from build123d import *

# Parameters (mm, degrees)
SKETCH1_R           = 1.6
BOSS_EXTRUDE1_DEPTH = 3
FILLET1_R           = 10
FILLET2_R           = 2
FILLET3_R           = 2


# Some blends are built 0.0001 mm under size
with BuildPart() as part:
    # Sketch1 → Boss-Extrude1 (new body)
    with BuildSketch(Plane.XY):
        with BuildLine():
            Line((-15, 37.5), (-11.986741947, -0.333454454))
            Line((-11.986741947, -0.333454454), (-11.77, -31.11))
            ThreePointArc((-11.77, -31.11), (-7.007950772, -32.588761506), (-3.921159912, -36.504827214))
            ThreePointArc((-3.921159912, -36.504827214), (0, -39.2), (3.921159912, -36.504827214))
            ThreePointArc((3.921159912, -36.504827214), (7.007950772, -32.588761506), (11.77, -31.11))
            Line((11.77, -31.11), (11.986741947, -0.333454454))
            Line((11.986741947, -0.333454454), (15, 37.5))
            Line((15, 37.5), (15, 62.5))
            ThreePointArc((15, 62.5), (14.0627417, 64.7627417), (11.8, 65.7))
            Line((11.8, 65.7), (-11.8, 65.7))
            ThreePointArc((-11.8, 65.7), (-14.0627417, 64.7627417), (-15, 62.5))
            Line((-15, 62.5), (-15, 37.5))
        make_face()
        with Locations((7.8, 0)):
            Circle(SKETCH1_R, mode=Mode.SUBTRACT)
        with Locations((-12, 37.5)):
            Circle(SKETCH1_R, mode=Mode.SUBTRACT)
        with Locations((-12, 62.5)):
            Circle(SKETCH1_R, mode=Mode.SUBTRACT)
        Polygon((-7.5, 57.5), (7.5, 57.5), (7.5, 52), (11.5, 52), (11.5, 48), (7.5, 48), (7.5, 42.5), (-7.5, 42.5), (-7.5, 48), (-11.5, 48), (-11.5, 52), (-7.5, 52), align=None, mode=Mode.SUBTRACT)
        with Locations((12, 37.5)):
            Circle(SKETCH1_R, mode=Mode.SUBTRACT)
        with Locations((12, 62.5)):
            Circle(SKETCH1_R, mode=Mode.SUBTRACT)
        with Locations((-7.8, 0)):
            Circle(SKETCH1_R, mode=Mode.SUBTRACT)
        with Locations((0, -35)):
            Circle(SKETCH1_R, mode=Mode.SUBTRACT)
    extrude(amount=BOSS_EXTRUDE1_DEPTH)

    # Fillet1
    # the kernel refuses this fillet: 10 mm, written as the material it adds along each edge
    with BuildSketch(Plane(origin=(-11.986741947, -0.333454454, 0), x_dir=(-0.07939391755808242, 0.9968433206150205, 0), z_dir=(0, 0, 1)), Plane(origin=(11.986741947, -0.333454454, 0), x_dir=(-0.0070422644314045895, -0.9999752029483923, 0), z_dir=(0, 0, 1))) as fillet1_piece_1:
        with BuildLine():
            CenterArc((FILLET1_R * 0.0362334645201, FILLET1_R), FILLET1_R, 265.849766407, 4.150233593)
            Line((-FILLET1_R * 0.0361384500424, FILLET1_R * 0.00262228519856), (0, 0))
            Line((0, 0), (FILLET1_R * 0.0362334645201, 0))
        make_face()
    extrude(amount=3)
    # the kernel refuses this fillet: 10 mm, written as the material it takes off along each edge
    with BuildSketch(Plane(origin=(-11.77, -31.11, -17.521148691), x_dir=(-0.007042264431403126, 0.9999752029483922, 0), z_dir=(0, 0, 1))) as fillet1_2_piece_1:
        with BuildLine():
            CenterArc((7.008459476, -10), FILLET1_R, 90, 56.873561784)
            ThreePointArc((-1.366206899, -4.535115453), (-0.357121593, -2.365760003), (0, 0))
            Line((0, 0), (7.008459476, 0))
        make_face()
    extrude(amount=38.042297381, mode=Mode.SUBTRACT)
    with BuildSketch(Plane(origin=(-15, 37.5, -0.993992828), x_dir=(0, 1, 0), z_dir=(0, 0, 1)), Plane(origin=(15, 37.5, -0.993992828), x_dir=(-0.07939391755808864, -0.9968433206150199, 0), z_dir=(0, 0, 1))) as fillet1_2_piece_2:
        with BuildLine():
            CenterArc((FILLET1_R * 0.0397597131124, -FILLET1_R), FILLET1_R, 90, 4.553728958)
            Line((-FILLET1_R * 0.0396342044457, -FILLET1_R * 0.00315667938498), (0, 0))
            Line((0, 0), (FILLET1_R * 0.0397597131124, 0))
        make_face()
    extrude(amount=4.987985656, mode=Mode.SUBTRACT)
    with BuildSketch(Plane(origin=(11.77, -31.11, -17.521148691), x_dir=(-0.9595036182786473, -0.2816963019107352, 0), z_dir=(0, 0, 1))) as fillet1_2_piece_3:
        with BuildLine():
            CenterArc((7.553395586, -9.595036183), FILLET1_R, 106.361471425, 56.873561784)
            Line((-2.02156487, -6.710572234), (0, 0))
            ThreePointArc((0, 0), (2.368216284, -0.34045243), (4.736432567, 0))
        make_face()
    extrude(amount=38.042297381, mode=Mode.SUBTRACT)

    # Fillet2
    fillet2_edges = [part.edges().sort_by_distance(p)[0] for p in [
        (-11.5, 52, 1.5),
        (-11.5, 48, 1.5),
    ]]
    fillet(fillet2_edges, radius=FILLET2_R - 0.0001)  # a hair under: the kernel refuses the full size

    # Fillet3
    fillet3_edges = [part.edges().sort_by_distance(p)[0] for p in [
        (11.5, 48, 1.5),
        (11.5, 52, 1.5),
    ]]
    fillet(fillet3_edges, radius=FILLET3_R - 0.0001)  # a hair under: the kernel refuses the full size


solid = part.part
Geometry: final body of the model. Coordinates: model frame, mm. A direction names the side the tool comes from. Give positions to 0.01 mm unless a question says otherwise; leave off trailing zeros. Write each loop counter-clockwise with the first axis right and the second up, starting at its lowest first coordinate (ties: lowest second). Pieces come first, ordered by that corner, then holes. Notation, with made-up numbers: M -25.5,-13.75 L -12.5,-13.75 A18 ccw -12.5,0.25 Z; hole C -25.75,-30 d11. An arc over 180 degrees is marked long. Answer in a Markdown table with one row per item. Add a question column.
(1) Section B-B on y = -35. Return loops of the section in (x, z).
(2) Reachability of faces 5 (the flat face through (13.47, 18.31, 1.48)), 6 (the cylindrical face through (-10.93, 51.4, 1.52)) from +Z, -Z, +X, -X, +Y, -Y: full face, straight path, thin tool, end or side. Return the list, or none.
(3) Mould query, pull axis X, two halves, no side actions, for faces 1 (the flat face through (-13.513, 18.825, 1.479)), 2 (the flat face through (2, 15, 3)), 3 (the cylindrical face through (9.28, -0.61, 1.48)), 4 (the flat face through (-8, 48, 1)). Classes: +X half, -X half, draft (parallel to the pull), parting line (faces both ways), or undercut.
(4) Ray query, line 1 (Y direction, x = 0, z = 1.25); line 2 (Y direction, x = -6, z = 2.85); line 3 (X direction, y = 56.5, z = 2.85). Return the intervals inside material, ascending.
(5) Section A-A on x = 0. Return loops of the section in (y, z).
(6) Section C-C on z = 0.85. State how many separate pieces and enclosed holes the cut face has, and give its area (3 significant figures).
(7) First-contact query: pin 1 (1 mm diameter, centred on x = -10.5, z = 1.5, fed in from -Y); pin 2 (1.5 mm diameter, centred on x = 1, z = 1.5, fed in from -Y); pin 3 (1.6 mm diameter, centred on x = 8, z = 1.5, fed in from -Y). Flat tips, straight axial feed; report the tip coordinate or a pass-through.
(8) Section D-D on y = 33.5. Return loops of the section in (x, z), and give its area (3 significant figures).
Result set:
| question | item | result |
|---|---|---|
| 1 | outline | M -4.68,0 L -1.6,0 L -1.6,3 L -4.68,3 Z; M 1.6,0 L 4.68,0 L 4.68,3 L 1.6,3 Z |
| 2 | face 5 | +Z, -Z, +X, -Y |
| 2 | face 6 | +Z, -Z |
| 3 | face 1 | -X half |
| 3 | face 2 | draft |
| 3 | face 3 | undercut |
| 3 | face 4 | undercut |
| 4 | line 1 | y = -39.2 to -36.6, -33.4 to 42.5, 57.5 to 65.7 |
| 4 | line 2 | y = -33.4 to 42.5, 57.5 to 65.7 |
| 4 | line 3 | x = -15 to -7.5, 7.5 to 15 |
| 5 | outline | M -39.2,0 L -36.6,0 L -36.6,3 L -39.2,3 Z; M -33.4,0 L 42.5,0 L 42.5,3 L -33.4,3 Z; M 57.5,0 L 65.7,0 L 65.7,3 L 57.5,3 Z |
| 6 | separate pieces | 1 |
| 6 | enclosed holes | 8 |
| 6 | area | 2,350 mm^2 |
| 7 | pin 1 | stops at y = -29.78 |
| 7 | pin 2 | stops at y = -39.19 |
| 7 | pin 3 | stops at y = -32.46 |
| 8 | outline | M -14.68,0 L 14.68,0 L 14.68,3 L -14.68,3 Z |
| 8 | area | 88.1 mm^2 |
